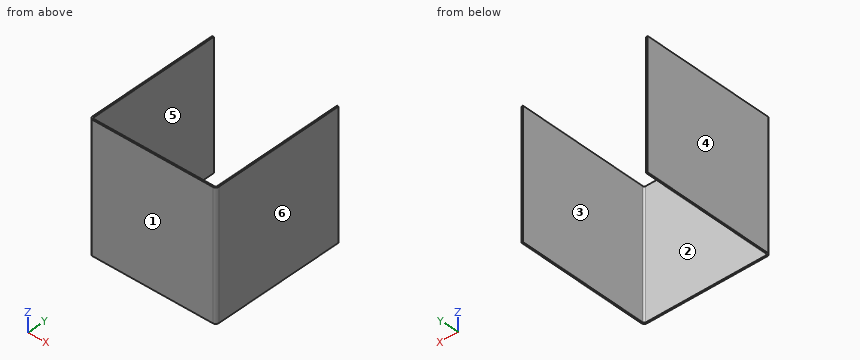
```python
from build123d import *

# Parameters (mm, degrees)
SKETCH002_W  = 248
SKETCH002_H  = 264
PAD002_DEPTH = 250
FILLET002_R  = 6
THICKNESS_T  = -3


with BuildPart() as part:
    # Sketch002 → Pad002 (new body)
    with BuildSketch(Plane.XY):
        with Locations((0, -132)):
            Rectangle(SKETCH002_W, SKETCH002_H)
    extrude(amount=PAD002_DEPTH)

    # Fillet002
    fillet002_edges = [part.edges().sort_by_distance(p)[0] for p in [
        (124, -264, 125),
        (-124, -264, 125),
    ]]
    fillet(fillet002_edges, radius=FILLET002_R)

    # Thickness
    thickness_openings = [part.faces().sort_by_distance(p)[0] for p in [
        (0, -131.969157, 250),
        (0, 0, 125),
        (0, -131.969157, 0),
    ]]
    offset(amount=THICKNESS_T, openings=thickness_openings)


solid = part.part
```
Geometry check sheet. Reference: the model listing, model coordinates, mm. Face numbers are marked on the shaded views. A direction names the side the tool comes from. Coordinates: 2 decimals unless noted, no trailing zeros. Loops run counter-clockwise (first coordinate to the right, second up) from the corner with the lowest first, then second, coordinate; pieces in that order, holes last.
Item 1: Sectioned sample at A-A, the plane y = -16.5. Record the boundary of the cut face in (x, z), then the cut area to 3 significant figures.
Item 2: Go/stop test with a flat-tipped pin: pin 1 Ø10 at (x, z) = (28, 107.5) entering from +Y. Record where the tip stops, or that it passes through.
Item 3: Sectioned sample at B-B, the plane z = 214.5. Record the boundary of the cut face in (x, y).
Item 4: Release check for a two-part mould opening along X. For the marked faces 3, 4, 5 and 6 record: released by +X, released by -X, zero draft, split by the parting line, or undercut.
Item 5: Access from +Z, -Z, +X, -X, +Y, -Y to the whole of each face (thin tool, end or side, straight path). Record for the marked faces 1 and 2.
Item 6: Thickness scan on line 1 (X direction, y = -201, z = 35); line 2 (Y direction, x = 89.5, z = 175). Record the ranges inside material, lowest first.
Item 7: Sectioned sample at C-C, the plane x = 79.5. Record the boundary of the cut face in (y, z), then the cut area to 3 significant figures.
Check result:
1. outline: (-124, 0) - (-121, 0) - (-121, 250) - (-124, 250) - close; (121, 0) - (124, 0) - (124, 250) - (121, 250) - close
1. area: 1,500 mm2
2. pin 1: stops at y = -261
3. outline: (-124, -258) arc R6 ccw to (-118, -264) - (118, -264) arc R6 ccw to (124, -258) - (124, 0) - (121, 0) - (121, -258) arc R3 cw to (118, -261) - (-118, -261) arc R3 cw to (-121, -258) - (-121, 0) - (-124, 0) - close
4. face 3: undercut
4. face 4: released by -X
4. face 5: undercut
4. face 6: released by +X
5. face 1: +Z, -Z, +X, -X, -Y
5. face 2: +Z, -Z, +Y
6. line 1: x = -124 to -121, 121 to 124
6. line 2: y = -264 to -261
7. outline: (-264, 0) - (-261, 0) - (-261, 250) - (-264, 250) - close
7. area: 750 mm2
